```python
from build123d import *
from build123d.topology import SkipClean

# Parameters (mm, degrees)
BASE_SKETCH_R                   = 30
BASE_EXTRUDE_DEPTH              = 30
PIN_SKETCH_R                    = 20
PIN_EXTRUDE_DEPTH               = 100
SIDE_CUT_REACH                  = 138.748
SIDE_CUT_END_RADIUS             = 30
SIDE_CUT_SKETCH_R               = 25
SIDE_CUT_DIRECTION_2_REACH      = 138.748
SIDE_CUT_DIRECTION_2_END_RADIUS = 30
WING_EXTRUDE_REACH              = 146.309
WING_EXTRUDE_END_RADIUS         = 30
PIN_HOLE_CUT_DEPTH              = 145.308696956
PIN_HOLE_CUT_DEPTH_BACK         = 145.308696956
PIN_HOLE_SKETCH_R               = 5


with BuildPart() as part:
    # Base Sketch → Base Extrude (new body)
    with BuildSketch(Plane.XY):
        Circle(BASE_SKETCH_R)
    extrude(amount=BASE_EXTRUDE_DEPTH)

    # Pin Sketch → Pin Extrude (add)
    with BuildSketch(Plane.XY.offset(30)):
        Circle(PIN_SKETCH_R)
    extrude(amount=PIN_EXTRUDE_DEPTH)

    # Side Cut: up to this cylinder (the profile starts inside it)
    side_cut_end = Plane(origin=(0, 0, 0), z_dir=(0, 0, -1)) * Cylinder(SIDE_CUT_END_RADIUS, 338.496, mode=Mode.PRIVATE)
    # Side Cut Sketch → Side Cut (cut, up to the surface)
    with BuildSketch(Plane(origin=(0, 0, 0), x_dir=(0, 0, -1), z_dir=(1, 0, 0)), mode=Mode.PRIVATE) as side_cut_sk1:
        Circle(SIDE_CUT_SKETCH_R)
    side_cut_tool1 = extrude(side_cut_sk1.sketch, amount=-SIDE_CUT_REACH, mode=Mode.PRIVATE) & side_cut_end
    add(side_cut_tool1.solids().sort_by_distance((0, 0, 0))[0], mode=Mode.SUBTRACT)

    # Side Cut direction 2: up to this cylinder (the profile starts inside it)
    side_cut_direction_2_end = Plane(origin=(0, 0, 0), z_dir=(0, 0, -1)) * Cylinder(SIDE_CUT_DIRECTION_2_END_RADIUS, 338.496, mode=Mode.PRIVATE)
    # Side Cut Sketch → Side Cut direction 2 (cut, up to the surface)
    with BuildSketch(Plane(origin=(0, 0, 0), x_dir=(0, 0, -1), z_dir=(1, 0, 0)), mode=Mode.PRIVATE) as side_cut_direction_2_sk1:
        Circle(SIDE_CUT_SKETCH_R)
    side_cut_direction_2_tool1 = extrude(side_cut_direction_2_sk1.sketch, amount=SIDE_CUT_DIRECTION_2_REACH, mode=Mode.PRIVATE) & side_cut_direction_2_end
    add(side_cut_direction_2_tool1.solids().sort_by_distance((0, 0, 0))[0], mode=Mode.SUBTRACT)

    # Wing Extrude: up to this cylinder (the profile starts inside it)
    with SkipClean():  # the faces are left unmerged after this step: merging them gives an invalid solid
        wing_extrude_end = Plane(origin=(0, 0, -18.188486), z_dir=(0, 0, -1)) * Cylinder(WING_EXTRUDE_END_RADIUS, 353.618, mode=Mode.PRIVATE)
        # Wing Sketch → Wing Extrude (add, up to the surface)
        with BuildSketch(Plane(origin=(0, 25, 0), x_dir=(1, 0, 0), z_dir=(0, 1, 0)), mode=Mode.PRIVATE) as wing_extrude_sk1:
            with BuildLine():
                Line((-16.583123952, 0), (-14.971098535, 25.930703308))
                ThreePointArc((-14.971098535, 25.930703308), (0, 40), (14.971098535, 25.930703308))
                Line((14.971098535, 25.930703308), (16.583123952, 0))
                Line((16.583123952, 0), (-16.583123952, 0))
            make_face()
        wing_extrude_tool1 = extrude(wing_extrude_sk1.sketch, amount=WING_EXTRUDE_REACH, mode=Mode.PRIVATE) & wing_extrude_end
        wing_extrude = wing_extrude_tool1.solids().sort_by_distance((0, 25, -18.188486))[0]
        add(wing_extrude)

    # Wing Mirror: Wing Extrude across plane
    with SkipClean():  # the faces are left unmerged after this step: merging them gives an invalid solid
        add(wing_extrude.mirror(Plane.ZX))

    # Pin Hole Sketch → Pin Hole Cut (cut, two sides: drawn at the far end of the back side and taken through both)
    with SkipClean():  # the faces are left unmerged after this step: merging them gives an invalid solid
        with BuildSketch(Plane.XZ.offset(-25).offset(-PIN_HOLE_CUT_DEPTH_BACK)):
            with Locations(Location((0, -25, 0), (0, 0, 90))):
                Circle(PIN_HOLE_SKETCH_R)
        extrude(amount=PIN_HOLE_CUT_DEPTH + PIN_HOLE_CUT_DEPTH_BACK, mode=Mode.SUBTRACT)


solid = part.part
```
Verification items for the finished model (mm, model axes). A direction names the side the tool comes from. Give positions to 0.01 mm unless a question says otherwise; leave off trailing zeros. Order: outer loops, then holes, each group sorted by start corner. A loop starts at its lowest first (then second) coordinate and runs counter-clockwise, first axis right, second up. Notation, with made-up numbers: (45.25, 40) -> (99.25, 40) arc R25 ccw to (99.25, 73) -> close; hole circle Ø6 at (-4, 89.25). An arc over 180 degrees is marked (long way). Use a Markdown table: item, result.
1) Material ranges on probe 1 along Z at (x, y) = (-4, 27); probe 2 along X at (y, z) = (-27, -25); probe 3 along X at (y, z) = (27.75, -25), recorded low to high.
Results:
| item | result |
|---|---|
| probe 1 | -39.46 to -28, -22 to 30 |
| probe 2 | -13.08 to -5, 5 to 13.08 |
| probe 3 | -11.4 to -5, 5 to 11.4 |
2) Mould release check, pull along X, two halves, no side actions. Record for faces 4 (the cylindrical face through (-4.336, -19.524, 79.3)), 5 (the flat face through (0, 0, 130)), 6 (the cylindrical face through (-4.957, -27.465, -25.651)): pulls with the +X half, pulls with the -X half, needs draft (parallel to the pull), parting line crosses it, or undercut.
Results:
| item | result |
|---|---|
| face 4 | parting line crosses it |
| face 5 | needs draft |
| face 6 | undercut |
3) Section check C-C, the plane y = 0. Record the boundary of the cut face in (x, z).
Results:
| item | result |
|---|---|
| outline | (-30, 25) -> (30, 25) -> (30, 30) -> (20, 30) -> (20, 130) -> (-20, 130) -> (-20, 30) -> (-30, 30) -> close |
4) Section check D-D, the plane z = 12.5. Record the boundary of the cut face in (x, y), then the cut area to 3 significant figures.
Results:
| item | result |
|---|---|
| outline | (-20.77, -21.65) arc R30 ccw to (20.77, -21.65) -> close; (-20.77, 21.65) -> (20.77, 21.65) arc R30 ccw to start |
| area | 477 mm² |
5) Tool access check on faces 1 (the flat face through (6, -20, 30)), 2 (the flat face through (0, -25, -16)), 3 (the cylindrical face through (0, 28, -30)). Record the directions out of +Z, -Z, +X, -X, +Y, -Y that give a thin tool (end or side, any length) a straight path to the whole face; none if there is none.
Results:
| item | result |
|---|---|
| face 1 | +Z |
| face 2 | -Z, +X, -X |
| face 3 | +Y, -Y |
6) Depth check by flat-ended pin: pin 1 Ø4 at (y, z) = (3, 43.5) entering from -X (3 decimals); pin 2 Ø2 at (x, z) = (-9, 85.5) entering from +Y; pin 3 Ø4 at (x, y) = (22.5, 21.5) entering from -Z. Enter the tip coordinate at first touch or a pass-through.
Results:
| item | result |
|---|---|
| pin 1 | x = -19.975 |
| pin 2 | y = 18.33 |
| pin 3 | z = 12.11 |
7) Section check A-A, the plane x = 0. Record the boundary of the cut face in (y, z).
Results:
| item | result |
|---|---|
| outline | (-30, -40) -> (-25, -40) -> (-25, -30) -> (-30, -30) -> close; (-30, -20) -> (-25, -20) -> (-25, 0) arc R25 cw to (25, 0) -> (25, -20) -> (30, -20) -> (30, 30) -> (20, 30) -> (20, 130) -> (-20, 130) -> (-20, 30) -> (-30, 30) -> close; (25, -40) -> (30, -40) -> (30, -30) -> (25, -30) -> close |
8) Section check B-B, the plane z = -28. Record the boundary of the cut face in (x, y), then the cut area to 3 significant figures.
Results:
| item | result |
|---|---|
| outline | (-14.7, -26.15) arc R30 ccw to (-4, -29.73) -> (-4, -25) -> (-14.7, -25) -> close; (-14.7, 25) -> (-4, 25) -> (-4, 29.73) arc R30 ccw to (-14.7, 26.15) -> close; (4, -29.73) arc R30 ccw to (14.7, -26.15) -> (14.7, -25) -> (4, -25) -> close; (4, 25) -> (14.7, 25) -> (14.7, 26.15) arc R30 ccw to (4, 29.73) -> close |
| area | 142 mm² |
